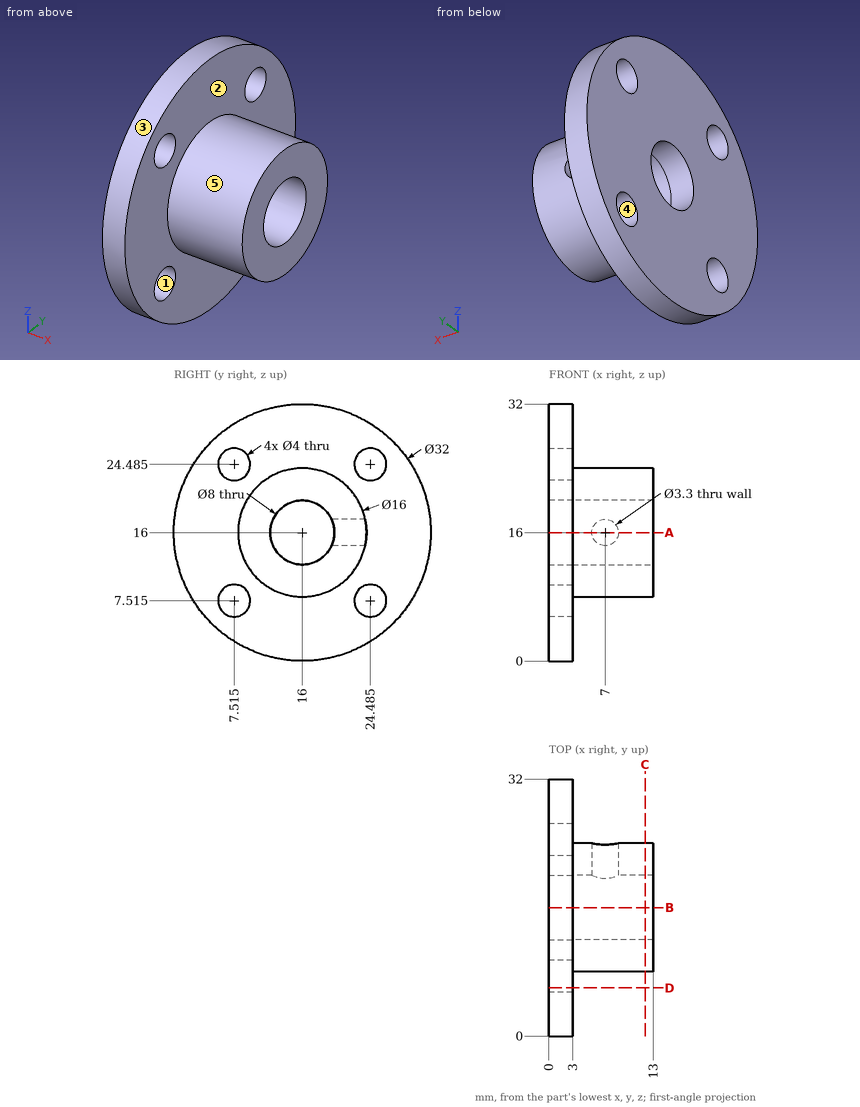
Source: three-view drawing plus pictorial views. Frame: mm from the lowest corner of the part. A direction names the side the tool comes from. Coordinates: 2 decimals unless noted, no trailing zeros. Write each loop counter-clockwise with the first axis right and the second up, starting at its lowest first coordinate (ties: lowest second). Pieces come first, ordered by that corner, then holes. Notation, with made-up numbers: (-13.75, 50) -> (39.25, 50) arc R17 cw to (39.25, 73) -> close; hole circle Ø2 at (18, 56.5). An arc over 180 degrees is marked (long way). Answer as a JSON object with one key per item and string values.
1. Mould query, pull axis Y, two halves, no side actions, for the marked faces 1, 2 and 3. Classes: released by +Y, released by -Y, zero draft, split by the parting line, or undercut.
Result set:
{"face 1": "undercut", "face 2": "zero draft", "face 3": "split by the parting line"}
2. Access query for the marked faces 4 and 5. Directions: +Z, -Z, +X, -X, +Y, -Y. A direction counts if a zero-diameter tool reaches every point of the face in a straight line with its end or side. Return the directions, or none.
Result set:
{"face 4": "+X, -X", "face 5": "+X"}
3. Section D-D on y = 6. Return the cut outline in (x, z).
Result set:
{"outline": "(0, 3.51) -> (3, 3.51) -> (3, 6.21) -> (0, 6.21) -> close; (0, 8.82) -> (3, 8.82) -> (3, 23.18) -> (0, 23.18) -> close; (0, 25.79) -> (3, 25.79) -> (3, 28.49) -> (0, 28.49) -> close"}
4. First-contact query: P1, Ø5, axis at x = 9, y = 25.5, coming from the +Z side (1 decimal); P2, Ø4, axis at x = 4, y = 25, coming from the -Z side (1 decimal); P3, Ø6, axis at x = 7.5, y = 8, coming from the +Z side (1 decimal). Flat tips, straight axial feed; report the tip coordinate or a pass-through.
Result set:
{"P1": "stops at z = 19.9", "P2": "stops at z = 1.7", "P3": "stops at z = 22.2"}
5. Section C-C on x = 12. Return the cut outline in (y, z), then the cut area to 3 significant figures.
Result set:
{"outline": "circle Ø16 at (16, 16); hole circle Ø8 at (16, 16)", "area": "151 mm2"}
6. Section B-B on y = 16. Return the cut outline in (x, z), then the cut area to 3 significant figures.
Result set:
{"outline": "(0, 0) -> (3, 0) -> (3, 8) -> (13, 8) -> (13, 12) -> (0, 12) -> close; (0, 20) -> (13, 20) -> (13, 24) -> (3, 24) -> (3, 32) -> (0, 32) -> close", "area": "152 mm2"}
7. Section A-A on z = 16. Return the cut outline in (x, y).
Result set:
{"outline": "(0, 0) -> (3, 0) -> (3, 8) -> (13, 8) -> (13, 12) -> (0, 12) -> close; (0, 20) -> (5.35, 20) -> (5.35, 24) -> (3, 24) -> (3, 32) -> (0, 32) -> close; (8.65, 20) -> (13, 20) -> (13, 24) -> (8.65, 24) -> close"}
8. Material intervals for line 1 (X direction, y = 21.5, z = 16); line 2 (Y direction, x = 1.15, z = 16); line 3 (Y direction, x = 2.5, z = 7.5) (1 decimal), sorted ascending. Write a range as from..to.
Result set:
{"line 1": "x = 0..5.35, 8.65..13", "line 2": "y = 0..12, 20..32", "line 3": "y = 2.4..5.5, 9.5..22.5, 26.5..29.6"}
